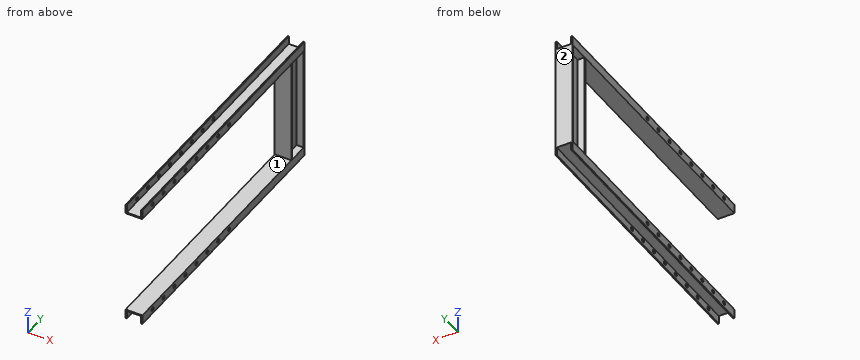
```python
from build123d import *

# Parameters (mm, degrees)
BOSS_EXTRUDE1_DEPTH     = 285.75
BOSS_EXTRUDE2_DEPTH     = 1504.95
SKETCH4_R               = 10.033
CUT_EXTRUDE1_DEPTH      = 1428.530782148
LPATTERN1_COUNT         = 8
LPATTERN1_PITCH         = 101.6
MIRROR2_COPY_1_SKETCH_R = 10.033
MIRROR2_COPY_1_DEPTH    = 1428.530782148
MIRROR2_COPY_2_SKETCH_R = 10.033
MIRROR2_COPY_2_DEPTH    = 1428.530782148
MIRROR2_COPY_3_SKETCH_R = 10.033
MIRROR2_COPY_3_DEPTH    = 1428.530782148
MIRROR2_COPY_4_SKETCH_R = 10.033
MIRROR2_COPY_4_DEPTH    = 1428.530782148
MIRROR2_COPY_5_SKETCH_R = 10.033
MIRROR2_COPY_5_DEPTH    = 1428.530782148
MIRROR2_COPY_6_SKETCH_R = 10.033
MIRROR2_COPY_6_DEPTH    = 1428.530782148
MIRROR2_COPY_7_SKETCH_R = 10.033
MIRROR2_COPY_7_DEPTH    = 1428.530782148


with BuildPart() as part:
    # Sketch1 → Boss-Extrude1 (new, symmetric)
    with BuildSketch(Plane.XY):
        Polygon((45.5295, 120.65), (45.5295, 114.3), (6.35, 114.3), (6.35, 6.35), (45.5295, 6.35), (45.5295, 0), (0, 0), (0, 120.65), align=None)
    boss_extrude1 = extrude(amount=BOSS_EXTRUDE1_DEPTH, both=True)

    # Mirror1: Boss-Extrude1 across plane
    add(boss_extrude1.mirror(Plane(origin=(0, 120.65, 285.75), x_dir=(0, 0, 1), z_dir=(1, 0, 0))))

    # Sketch3 → Boss-Extrude2 (add)
    with BuildSketch(Plane(origin=(0, 120.65, 0), x_dir=(1, 0, 0), z_dir=(0, 1, 0))):
        Polygon((-45.5295, -285.75), (45.5295, -285.75), (45.5295, -336.55), (39.1795, -336.55), (39.1795, -292.1), (-39.1795, -292.1), (-39.1795, -336.55), (-45.5295, -336.55), align=None)
    boss_extrude2 = extrude(amount=-BOSS_EXTRUDE2_DEPTH)

    # Sketch4 → Cut-Extrude1 (cut, through all)
    with BuildSketch(Plane(origin=(45.5295, 0, 0), x_dir=(0, 0, -1), z_dir=(1, 0, 0))):
        with Locations((-311.15, -577.85)):
            Circle(SKETCH4_R)
    cut_extrude1 = extrude(amount=-CUT_EXTRUDE1_DEPTH, mode=Mode.SUBTRACT)

    # LPattern1: Cut-Extrude1 ×8
    with Locations(*[(0, -i * LPATTERN1_PITCH, 0) for i in range(1, LPATTERN1_COUNT)]):
        add(cut_extrude1, mode=Mode.SUBTRACT)

    # Mirror2: Boss-Extrude2, Cut-Extrude1 across plane
    add(boss_extrude2.mirror(Plane.XY))
    add(cut_extrude1.mirror(Plane.XY), mode=Mode.SUBTRACT)

    # Mirror2 copy 1 sketch → Mirror2 copy 1 (cut, through all)
    with BuildSketch(Plane(origin=(45.5295, -101.6, 0), x_dir=(0, 0, 1), z_dir=(1, 0, 0))):
        with Locations((-311.15, 577.85)):
            Circle(MIRROR2_COPY_1_SKETCH_R)
    extrude(amount=-MIRROR2_COPY_1_DEPTH, mode=Mode.SUBTRACT)

    # Mirror2 copy 2 sketch → Mirror2 copy 2 (cut, through all)
    with BuildSketch(Plane(origin=(45.5295, -203.2, 0), x_dir=(0, 0, 1), z_dir=(1, 0, 0))):
        with Locations((-311.15, 577.85)):
            Circle(MIRROR2_COPY_2_SKETCH_R)
    extrude(amount=-MIRROR2_COPY_2_DEPTH, mode=Mode.SUBTRACT)

    # Mirror2 copy 3 sketch → Mirror2 copy 3 (cut, through all)
    with BuildSketch(Plane(origin=(45.5295, -304.8, 0), x_dir=(0, 0, 1), z_dir=(1, 0, 0))):
        with Locations((-311.15, 577.85)):
            Circle(MIRROR2_COPY_3_SKETCH_R)
    extrude(amount=-MIRROR2_COPY_3_DEPTH, mode=Mode.SUBTRACT)

    # Mirror2 copy 4 sketch → Mirror2 copy 4 (cut, through all)
    with BuildSketch(Plane(origin=(45.5295, -406.4, 0), x_dir=(0, 0, 1), z_dir=(1, 0, 0))):
        with Locations((-311.15, 577.85)):
            Circle(MIRROR2_COPY_4_SKETCH_R)
    extrude(amount=-MIRROR2_COPY_4_DEPTH, mode=Mode.SUBTRACT)

    # Mirror2 copy 5 sketch → Mirror2 copy 5 (cut, through all)
    with BuildSketch(Plane(origin=(45.5295, -508, 0), x_dir=(0, 0, 1), z_dir=(1, 0, 0))):
        with Locations((-311.15, 577.85)):
            Circle(MIRROR2_COPY_5_SKETCH_R)
    extrude(amount=-MIRROR2_COPY_5_DEPTH, mode=Mode.SUBTRACT)

    # Mirror2 copy 6 sketch → Mirror2 copy 6 (cut, through all)
    with BuildSketch(Plane(origin=(45.5295, -609.6, 0), x_dir=(0, 0, 1), z_dir=(1, 0, 0))):
        with Locations((-311.15, 577.85)):
            Circle(MIRROR2_COPY_6_SKETCH_R)
    extrude(amount=-MIRROR2_COPY_6_DEPTH, mode=Mode.SUBTRACT)

    # Mirror2 copy 7 sketch → Mirror2 copy 7 (cut, through all)
    with BuildSketch(Plane(origin=(45.5295, -711.2, 0), x_dir=(0, 0, 1), z_dir=(1, 0, 0))):
        with Locations((-311.15, 577.85)):
            Circle(MIRROR2_COPY_7_SKETCH_R)
    extrude(amount=-MIRROR2_COPY_7_DEPTH, mode=Mode.SUBTRACT)


solid = part.part
```
Read the model definition and answer for the solid it produces. Units are mm, in the model's axes. Face numbers are marked on the shaded views. Round coordinates to 2 decimals unless told otherwise and drop trailing zeros. Loops run counter-clockwise (first coordinate to the right, second up) from the corner with the lowest first, then second, coordinate; pieces in that order, holes last. Notation, with made-up numbers: (-7.75, -22) -> (33.25, -22) arc R10 cw to (33.25, -17) -> close; hole circle Ø3 at (-14, -31.5). An arc over 180 degrees is marked (long way). One line per item, written item: value.
1) The mould has two halves that part along Z. Classify the marked faces 1 and 2: pulls with the +Z half, pulls with the -Z half, needs draft (parallel to the pull), parting line crosses it, or undercut.
Answer list:
face 1: undercut
face 2: needs draft
2) A cutting plane is placed at A-A (x = 23.5). Determine the outline of the cut face in (y, z), and give its area (3 significant figures).
Answer list:
outline: (-1384.3, -292.1) -> (120.65, -292.1) -> (120.65, 292.1) -> (-1384.3, 292.1) -> (-1384.3, 285.75) -> (0, 285.75) -> (0, -285.75) -> (-1384.3, -285.75) -> close; hole (6.35, -285.75) -> (114.3, -285.75) -> (114.3, 285.75) -> (6.35, 285.75) -> close
area: 26,400 mm²
3) Consider L1, parallel to Z at x = -41.25, y = -781.05; L2, parallel to Y at x = -28.5, z = -29.5; L3, parallel to Z at x = -32.5, y = -371. Determine where each line is inside the solid, lowest interval first. Write a range as [from, to].
Answer list:
L1: z = [-336.55, -321.18], [-301.12, -285.75], [285.75, 301.12], [321.18, 336.55]
L2: y = [0, 6.35], [114.3, 120.65]
L3: z = [-292.1, -285.75], [285.75, 292.1]
4) A cutting plane is placed at B-B (y = -264). Determine the outline of the cut face in (x, z), and give its area (3 significant figures).
Answer list:
outline: (-45.53, -336.55) -> (-39.18, -336.55) -> (-39.18, -292.1) -> (39.18, -292.1) -> (39.18, -336.55) -> (45.53, -336.55) -> (45.53, -285.75) -> (-45.53, -285.75) -> close; (-45.53, 285.75) -> (45.53, 285.75) -> (45.53, 336.55) -> (39.18, 336.55) -> (39.18, 292.1) -> (-39.18, 292.1) -> (-39.18, 336.55) -> (-45.53, 336.55) -> close
area: 2,290 mm²
5) A cutting plane is placed at C-C (z = -161.5). Determine the outline of the cut face in (x, y), and give its area (3 significant figures).
Answer list:
outline: (-45.53, 0) -> (45.53, 0) -> (45.53, 6.35) -> (6.35, 6.35) -> (6.35, 114.3) -> (45.53, 114.3) -> (45.53, 120.65) -> (-45.53, 120.65) -> (-45.53, 114.3) -> (-6.35, 114.3) -> (-6.35, 6.35) -> (-45.53, 6.35) -> close
area: 2,530 mm²
6) Flat-ended cylindrical pins translate along their axes: P1, Ø19.5, axis at x = -30, y = 56.5, coming from the -Z side; P2, Ø5, axis at x = 21.5, y = -459, coming from the +Z side; P3, Ø18, axis at y = -882.65, z = 311.15, coming from the +X side; P4, Ø12, axis at x = -24.5, y = -37.5, coming from the -Z side. Find the tip coordinate at first contact, or state that the pin passes through.
Answer list:
P1: stops at z = -336.55
P2: stops at z = 292.1
P3: passes through
P4: stops at z = -292.1
